Here's how the part is built. I have some questions about the finished solid (model axes, mm). Round coordinates to 2 decimals unless told otherwise and drop trailing zeros. Loops run counter-clockwise (first coordinate to the right, second up) from the corner with the lowest first, then second, coordinate; pieces in that order, holes last. Notation, with made-up numbers: M 12,-25.5 L 42,-25.5 A26 cw 42,-10.5 Z; hole C 62.25,78.25 d5. An arc over 180 degrees is marked long. Use a Markdown table: item, result.
from build123d import *

# Parameters (mm, degrees)
SKETCH2_W           = 73.66
SKETCH2_H           = 24.765
SKETCH2_W_2         = 5.08
SKETCH2_H_2         = 3.175
BOSS_EXTRUDE1_DEPTH = 3.175


with BuildPart() as part:
    # Sketch2 → Boss-Extrude1 (new body)
    with BuildSketch(Plane(origin=(0, 0, 0), x_dir=(1, 0, 0), z_dir=(0, 1, 0))):
        with Locations((0, -12.3825)):
            Rectangle(SKETCH2_W, SKETCH2_H)
        with Locations((-2.54, 1.5875)):
            Rectangle(SKETCH2_W_2, SKETCH2_H_2)
    extrude(amount=BOSS_EXTRUDE1_DEPTH)


solid = part.part
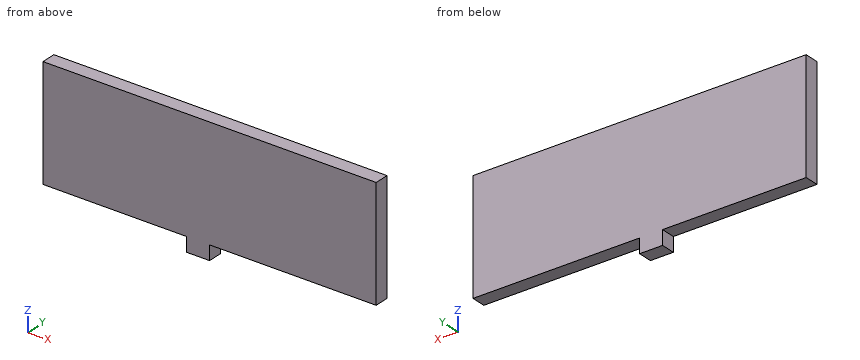
1. For pin 1 Ø1 at (y, z) = (1, -2.5) entering from +X; pin 2 Ø1.6 at (y, z) = (1, -2) entering from -X; pin 3 Ø10 at (x, z) = (16, 3) entering from -Y, each with a flat end and sliding along its axis, tell me the tip position at first contact or that it passes through.
Answer sheet:
| item | result |
|---|---|
| pin 1 | x = 0 |
| pin 2 | x = -5.08 |
| pin 3 | y = 0 |
2. I need wall thicknesses on probe 1 along Z at (x, y) = (5.5, 2.5) (3 decimals). Which ranges of the line are inside material? Lowest first, please. Write a range as from..to.
Answer sheet:
| item | result |
|---|---|
| probe 1 | 0..24.765 |
3. Imagine slicing it at A-A, the plane y = 0.8. Write out the boundary of the cut face in (x, z) (3 decimals).
Answer sheet:
| item | result |
|---|---|
| outline | M -36.83,0 L -5.08,0 L -5.08,-3.175 L 0,-3.175 L 0,0 L 36.83,0 L 36.83,24.765 L -36.83,24.765 Z |
4. Imagine slicing it at B-B, the plane x = 21.5. Write out the boundary of the cut face in (y, z) (3 decimals), then the cut area to 3 significant figures.
Answer sheet:
| item | result |
|---|---|
| outline | M 0,0 L 3.175,0 L 3.175,24.765 L 0,24.765 Z |
| area | 78.6 mm2 |
